The listing builds one solid part. Answer for the finished solid, in the listing's coordinates (mm). Face numbers are marked on the shaded views. Round coordinates to 2 decimals unless told otherwise and drop trailing zeros. Loops run counter-clockwise (first coordinate to the right, second up) from the corner with the lowest first, then second, coordinate; pieces in that order, holes last. Notation, with made-up numbers: M 1,8.5 L 53,8.5 A21 ccw 53,47.5 Z; hole C 73,83 d3. An arc over 180 degrees is marked long. Answer as a JSON object with one key per item and string values.
```python
from build123d import *

# Parameters (mm, degrees)
F0_R     = 17.5
F0_R_2   = 16
F1_DEPTH = 10
F2_W     = 5.6790858507
F2_H     = 2.5240386603
F2_H_2   = 1.5144229401
F2_H_3   = 1.0096157202
F3_DEPTH = 25


with BuildPart() as f1:
    # F0 (on Top) → F1 (new body)
    with BuildSketch(Plane.XY):
        Circle(F0_R)
        Circle(F0_R_2, mode=Mode.SUBTRACT)
    extrude(amount=F1_DEPTH)

    # F2 (on Right) → F3 (cut)
    with BuildSketch(Plane.YZ):
        with Locations((-0.0582132488, 6.4953924739)):
            Rectangle(F2_W, F2_H)
        with Locations((-0.0582132488, 3.4665459534)):
            Rectangle(F2_W, F2_H_2)
        with Locations((-0.0582132488, 4.7285652836)):
            Rectangle(F2_W, F2_H_3)
    extrude(amount=-F3_DEPTH, mode=Mode.SUBTRACT)


solid = f1.part
```
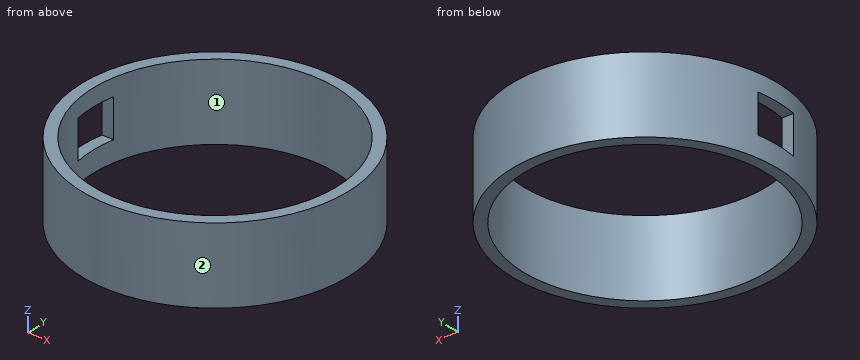
Item 1: Determine the mould class of the marked faces 1 and 2 for opening direction Y: released by +Y, released by -Y, zero draft, split by the parting line, or undercut.
Values follow:
{"face 1": "undercut", "face 2": "split by the parting line"}
Item 2: Flat-ended cylindrical pins translate along their axes: P1, Ø1.7, axis at x = -16.5, z = 4.5, coming from the +Y side; P2, Ø2, axis at y = -8.5, z = 6.5, coming from the -X side; P3, Ø1.7, axis at x = -16.5, z = 4, coming from the -Y side. Find the tip coordinate at first contact, or state that the pin passes through.
Values follow:
{"P1": "y = 7.83", "P2": "x = -15.81", "P3": "y = -7.83"}
Item 3: The part is cut by section C-C (y = 5). Give the vertices of the cut face in (x, z), then the cut area to 3 significant figures.
Values follow:
{"outline": "M -16.77,0 L -15.2,0 L -15.2,10 L -16.77,10 Z; M 15.2,0 L 16.77,0 L 16.77,10 L 15.2,10 Z", "area": "31.4 mm^2"}
Item 4: The part is cut by section B-B (y = 0). Give the vertices of the cut face in (x, z).
Values follow:
{"outline": "M -17.5,0 L -16,0 L -16,2.71 L -17.5,2.71 Z; M -17.5,7.76 L -16,7.76 L -16,10 L -17.5,10 Z; M 16,0 L 17.5,0 L 17.5,10 L 16,10 Z"}
Item 5: The part is cut by section A-A (x = 0). Give the vertices of the cut face in (y, z), then the cut area to 3 significant figures.
Values follow:
{"outline": "M -17.5,0 L -16,0 L -16,10 L -17.5,10 Z; M 16,0 L 17.5,0 L 17.5,10 L 16,10 Z", "area": "30.0 mm^2"}
Item 6: Straight lines are drawn through the part: line 1 (Y direction, x = 0, z = 6); line 2 (X direction, y = 0, z = 7); line 3 (Y direction, x = -4, z = 6.5). For each, find the intervals that lie inside material, in ascending order.
Values follow:
{"line 1": "-17.5 to -16, 16 to 17.5", "line 2": "16 to 17.5", "line 3": "-17.04 to -15.49, 15.49 to 17.04"}
Item 7: The part is cut by section D-D (z = 4). Give the vertices of the cut face in (x, y), then the cut area to 3 significant figures.
Values follow:
{"outline": "M -17.28,2.78 L -15.76,2.78 A16 cw long -15.74,-2.9 L -17.26,-2.9 A17.5 ccw long Z", "area": "149 mm^2"}
